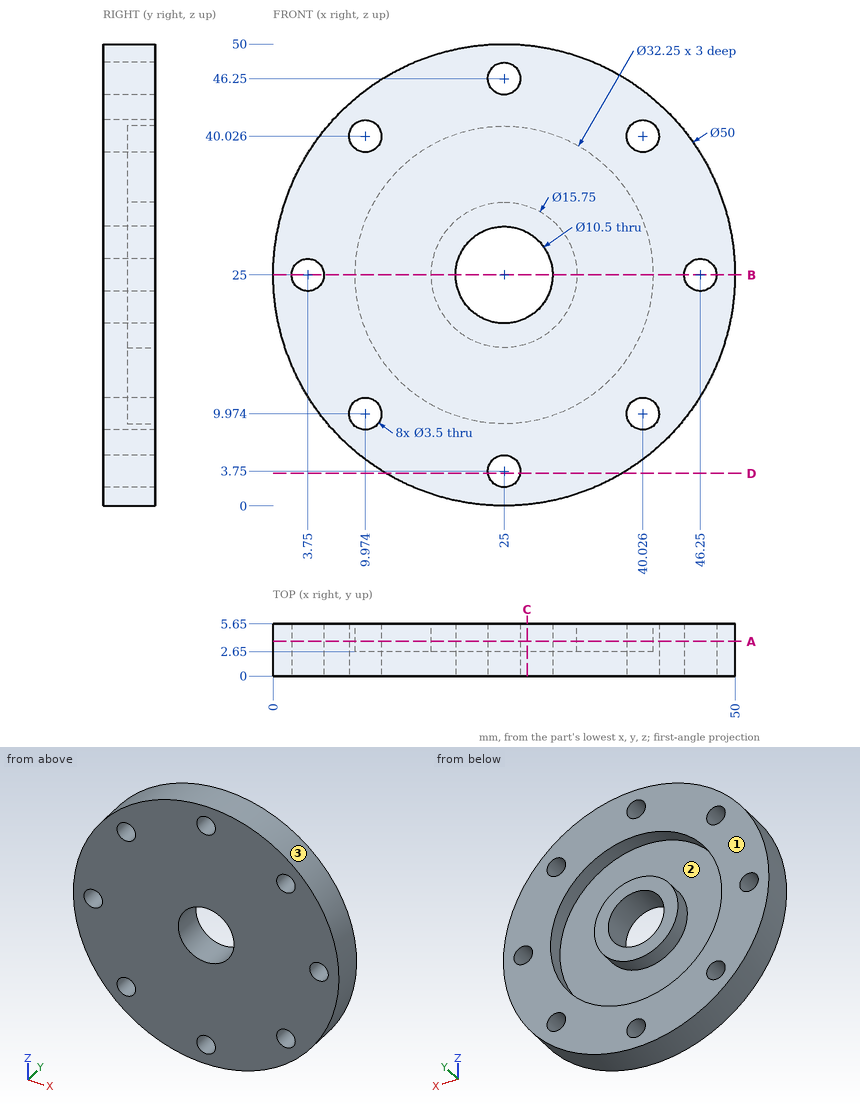
Answer from the drawing. Dimensions are ordinates in mm from the lowest x, y and z of the part. Give positions to 0.01 mm unless a question says otherwise; leave off trailing zeros. Write each loop counter-clockwise with the first axis right and the second up, starting at its lowest first coordinate (ties: lowest second). Pieces come first, ordered by that corner, then holes. Notation, with made-up numbers: (-6, -3) - (29, -3) arc R29 ccw to (29, 21) - close; hole circle Ø2 at (34, 20.25). An arc over 180 degrees is marked (long way). Answer in a Markdown table with one row per item. Add a question column.
Item 1: Find the intervals of material crossed by L1, parallel to X at y = 1.25, z = 25; L2, parallel to Z at x = 24, y = 3.15; L3, parallel to X at y = 1.2, z = 40.5 (1 decimal), in increasing order.
Item 2: Section D-D, the plane z = 3.5 is taken. Write down the section's boundary in (x, y).
Item 3: Section B-B, the plane z = 25 is taken. Write down the section's boundary in (x, y) (3 decimals).
Item 4: Section A-A, the plane y = 3.75 is taken. Count the separate pieces of the cut face and the enclosed holes in it, and give its area (3 significant figures).
Item 5: Section C-C, the plane x = 27.5 is taken. Write down the section's boundary in (y, z), and give its area (3 significant figures).
Item 6: Flat-ended cylindrical pins translate along their axes: P1, Ø1.5, axis at y = 3.5, z = 39.5, coming from the +X side; P2, Ø1.5, axis at x = 29.5, z = 14.5, coming from the +Y side; P3, Ø9.5, axis at x = 25, z = 25, coming from the +Y side; P4, Ø1.5, axis at y = 2, z = 37.5, coming from the +X side. Find the tip coordinate at first contact, or state that the pin passes through.
Item 7: Determine the mould class of the marked faces 1, 2 and 3 for opening direction X: pulls with the +X half, pulls with the -X half, needs draft (parallel to the pull), parting line crosses it, or undercut.
Recorded:
| question | item | result |
|---|---|---|
| 1 | L1 | x = 0 to 2, 5.5 to 19.75, 30.25 to 44.5, 48 to 50 |
| 1 | L2 | z = 0.02 to 2.31, 5.19 to 8.91, 17.19 to 19.85, 30.15 to 32.81, 41.09 to 44.81, 47.69 to 49.98 |
| 1 | L3 | x = 5.4 to 8.3, 11.7 to 38.3, 41.7 to 44.6 |
| 2 | outline | (12.24, 0) - (23.27, 0) - (23.27, 5.65) - (12.24, 5.65) - close; (26.73, 0) - (37.76, 0) - (37.76, 5.65) - (26.73, 5.65) - close |
| 3 | outline | (0, 0) - (2, 0) - (2, 5.65) - (0, 5.65) - close; (5.5, 0) - (19.75, 0) - (19.75, 5.65) - (17.125, 5.65) - (17.125, 2.65) - (8.875, 2.65) - (8.875, 5.65) - (5.5, 5.65) - close; (30.25, 0) - (44.5, 0) - (44.5, 5.65) - (41.125, 5.65) - (41.125, 2.65) - (32.875, 2.65) - (32.875, 5.65) - (30.25, 5.65) - close; (48, 0) - (50, 0) - (50, 5.65) - (48, 5.65) - close |
| 4 | separate pieces | 2 |
| 4 | enclosed holes | 10 |
| 4 | area | 1,180 mm2 |
| 5 | outline | (0, 0.13) - (5.65, 0.13) - (5.65, 9.07) - (2.65, 9.07) - (2.65, 17.53) - (5.65, 17.53) - (5.65, 20.38) - (0, 20.38) - close; (0, 29.62) - (5.65, 29.62) - (5.65, 32.47) - (2.65, 32.47) - (2.65, 40.93) - (5.65, 40.93) - (5.65, 49.87) - (0, 49.87) - close |
| 5 | area | 178 mm2 |
| 6 | P1 | stops at x = 45.88 |
| 6 | P2 | stops at y = 2.65 |
| 6 | P3 | passes through |
| 6 | P4 | stops at x = 47.07 |
| 7 | face 1 | needs draft |
| 7 | face 2 | undercut |
| 7 | face 3 | parting line crosses it |
